from build123d import *

# Parameters (mm, degrees)
F0_W     = 88.9
F0_H     = 63.5
F1_DEPTH = 6.35
F2_R     = 2.54
F4_DEPTH = 2
F6_DEPTH = 1.6256


with BuildPart() as f1:
    # F0 (on Top) → F1 (new body)
    with BuildSketch(Plane.XY):
        Rectangle(F0_W, F0_H)
    extrude(amount=F1_DEPTH)

    # F2
    f2_edges = [f1.edges().sort_by_distance(p)[0] for p in [
        (-44.45, -31.75, 3.175),
        (44.45, -31.75, 3.175),
        (44.45, 31.75, 3.175),
        (-44.45, 31.75, 3.175),
    ]]
    fillet(f2_edges, radius=F2_R)

    # F3 (on face) → F4 (cut)
    with BuildSketch(Plane.XY.offset(6.35)):
        with BuildLine():
            Line((38.735, 28.575), (-38.735, 28.575))
            ThreePointArc((-38.735, 28.575), (-40.531051, 27.831051), (-41.275, 26.035))
            Line((-41.275, 26.035), (-41.275, -26.035))
            ThreePointArc((-41.275, -26.035), (-40.531051, -27.831051), (-38.735, -28.575))
            Line((-38.735, -28.575), (38.735, -28.575))
            ThreePointArc((38.735, -28.575), (40.531051, -27.831051), (41.275, -26.035))
            Line((41.275, -26.035), (41.275, 26.035))
            ThreePointArc((41.275, 26.035), (40.531051, 27.831051), (38.735, 28.575))
        make_face()
    extrude(amount=-F4_DEPTH, mode=Mode.SUBTRACT)

    # F5 (on face) → F6 (cut)
    with BuildSketch(Plane.XY.offset(4.35)):
        with BuildLine():
            Line((35.814, 25.654), (-35.814, 25.654))
            ThreePointArc((-35.814, 25.654), (-37.610051, 24.910051), (-38.354, 23.114))
            Line((-38.354, 23.114), (-38.354, -23.114))
            ThreePointArc((-38.354, -23.114), (-37.610051, -24.910051), (-35.814, -25.654))
            Line((-35.814, -25.654), (35.814, -25.654))
            ThreePointArc((35.814, -25.654), (37.610051, -24.910051), (38.354, -23.114))
            Line((38.354, -23.114), (38.354, 23.114))
            ThreePointArc((38.354, 23.114), (37.610051, 24.910051), (35.814, 25.654))
        make_face()
    extrude(amount=-F6_DEPTH, mode=Mode.SUBTRACT)


solid = f1.part
Could you check a few things on this model? Use its own coordinates, in mm. A direction names the side the tool comes from. Give positions to 0.01 mm unless a question says otherwise; leave off trailing zeros. Write each loop counter-clockwise with the first axis right and the second up, starting at its lowest first coordinate (ties: lowest second). Pieces come first, ordered by that corner, then holes. Notation, with made-up numbers: (39, -39.75) -> (57, -39.75) arc R26 ccw to (57, -0.75) -> close; hole circle Ø9 at (47.5, 61). An arc over 180 degrees is marked (long way). Answer as a JSON object with one key per item and string values.
Q1. Suppose I cut it at A-A on y = -20. Write out the boundary of the cut face in (x, z) (3 decimals).
Taken from the geometry:
{"outline": "(-44.45, 0) -> (44.45, 0) -> (44.45, 6.35) -> (41.275, 6.35) -> (41.275, 4.35) -> (38.354, 4.35) -> (38.354, 2.724) -> (-38.354, 2.724) -> (-38.354, 4.35) -> (-41.275, 4.35) -> (-41.275, 6.35) -> (-44.45, 6.35) -> close"}
Q2. Suppose I cut it at B-B on x = -25. Write out the boundary of the cut face in (y, z) (3 decimals), then the cut area to 3 significant figures.
Taken from the geometry:
{"outline": "(-31.75, 0) -> (31.75, 0) -> (31.75, 6.35) -> (28.575, 6.35) -> (28.575, 4.35) -> (25.654, 4.35) -> (25.654, 2.724) -> (-25.654, 2.724) -> (-25.654, 4.35) -> (-28.575, 4.35) -> (-28.575, 6.35) -> (-31.75, 6.35) -> close", "area": "206 mm²"}
Q3. Please list where these lines run through material, in increasing order: L1, parallel to Y at x = 35, z = 3.25; L2, parallel to X at y = 6, z = 6 (3 decimals); L3, parallel to Y at x = -37, z = 5.25 (3 decimals).
Taken from the geometry:
{"L1": "y = -31.75 to -25.65, 25.65 to 31.75", "L2": "x = -44.45 to -41.275, 41.275 to 44.45", "L3": "y = -31.75 to -28.575, 28.575 to 31.75"}
Q4. We'd pull the mould along X, two halves only. Please class faces 1 (the flat face through (-41.275, 0, 5)), 2 (the cylindrical face through (-43.726, 30.986, 3.219)), 3 (the cylindrical face through (43.686, -31.026, 3.219)), 4 (the flat face through (-1, 0, 0)): released by +X, released by -X, zero draft, split by the parting line, or undercut.
Taken from the geometry:
{"face 1": "undercut", "face 2": "released by -X", "face 3": "released by +X", "face 4": "zero draft"}
Q5. Which directions (+Z, -Z, +X, -X, +Y, -Y) give clear straight access to the entire face, cutting with the end or side of a thin tool? Please do faces 5 (the flat face through (-1, -28.575, 5)), 6 (the flat face through (-4, -30, 6.35)).
Taken from the geometry:
{"face 5": "+Z", "face 6": "+Z, +X, -X, +Y, -Y"}
